Part print with two shaded views. Sizes in mm from the minimum x, y, z corner. A direction names the side the tool comes from. Give positions to 0.01 mm unless a question says otherwise; leave off trailing zeros. Order: outer loops, then holes, each group sorted by start corner. A loop starts at its lowest first (then second) coordinate and runs counter-clockwise, first axis right, second up. Notation, with made-up numbers: M 59.5,-0.5 L 68.5,-0.5 A4 ccw 68.5,3.5 Z; hole C -18,-8.5 d5. An arc over 180 degrees is marked long. Answer as CSV lines item,"result".
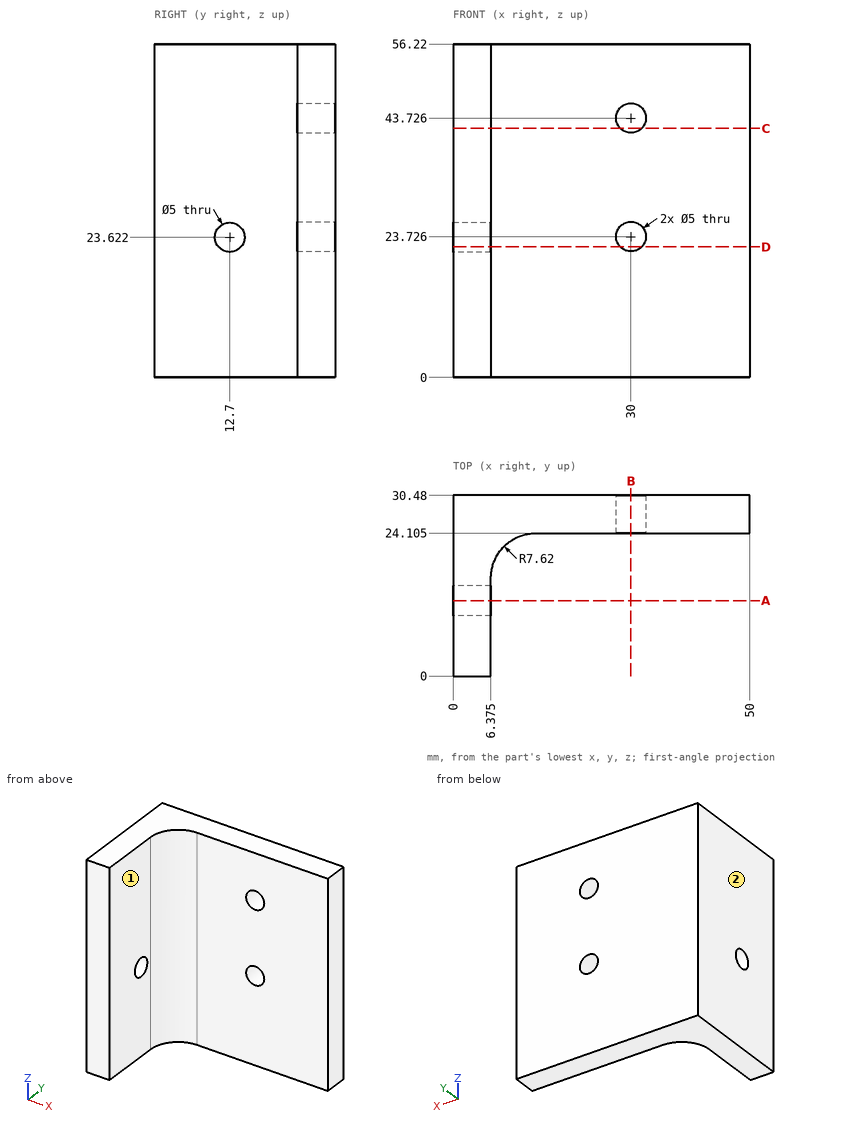
Item 1: Probe line 1 along Z through (x, y) = (30, 26); line 2 along Y through (x, z) = (33, 49.5) (1 decimal); line 3 along X through (y, z) = (12.5, 13.5) (1 decimal). List the from-to ranges inside material, lowest first. Write a range as from..to.
Geometry says:
line 1,"z = 0..21.23, 26.23..41.23, 46.23..56.22"
line 2,"y = 24.1..30.5"
line 3,"x = 0..6.4"
Item 2: Band-saw the part on C-C (z = 42). Give the cut face in (x, y) (1 decimal).
Geometry says:
outline,"M 0,0 L 6.4,0 L 6.4,16.5 A7.6 cw 14,24.1 L 28.2,24.1 L 28.2,30.5 L 0,30.5 Z; M 31.8,24.1 L 50,24.1 L 50,30.5 L 31.8,30.5 Z"
Item 3: 3-axis set-ups, long thin cutter, end or side, ignore diameter. For the marked faces 1 and 2: which of +Z, -Z, +X, -X, +Y, -Y reach the whole face in a straight line?
Geometry says:
face 1,"+Z, -Z, +X, -Y"
face 2,"+Z, -Z, -X, +Y, -Y"
Item 4: Band-saw the part on D-D (z = 22). Give the cut face in (x, y) (1 decimal).
Geometry says:
outline,"M 0,0 L 6.4,0 L 6.4,10.8 L 0,10.8 Z; M 0,14.6 L 6.4,14.6 L 6.4,16.5 A7.6 cw 14,24.1 L 28.2,24.1 L 28.2,30.5 L 0,30.5 Z; M 31.8,24.1 L 50,24.1 L 50,30.5 L 31.8,30.5 Z"
Item 5: Band-saw the part on B-B (x = 30). Give the cut face in (y, z) (1 decimal), and give its area (3 significant figures).
Geometry says:
outline,"M 24.1,0 L 30.5,0 L 30.5,21.2 L 24.1,21.2 Z; M 24.1,26.2 L 30.5,26.2 L 30.5,41.2 L 24.1,41.2 Z; M 24.1,46.2 L 30.5,46.2 L 30.5,56.2 L 24.1,56.2 Z"
area,"295 mm2"
Item 6: Band-saw the part on A-A (y = 12.7). Give the cut face in (x, z) (1 decimal).
Geometry says:
outline,"M 0,0 L 6.4,0 L 6.4,21.1 L 0,21.1 Z; M 0,26.1 L 6.4,26.1 L 6.4,56.2 L 0,56.2 Z"
Item 7: Drop flat-ended pins along their axis: pin 1 (4 mm diameter, centred on y = 12.7, z = 23.622, fed in from +X); pin 2 (6 mm diameter, centred on y = 16, z = 45, fed in from +X); pin 3 (4 mm diameter, centred on x = 21, z = 41, fed in from -Y) (1 decimal); pin 4 (1 mm diameter, centred on y = 4.5, z = 26, fed in from +X) (1 decimal). Give the stop position or say it passes through.
Geometry says:
pin 1,"passes through"
pin 2,"stops at x = 6.8"
pin 3,"stops at y = 24.1"
pin 4,"stops at x = 6.4"
